Could you check a few things on this model? Use its own coordinates, in mm. Face numbers are marked on the shaded views. A direction names the side the tool comes from. Coordinates: 2 decimals unless noted, no trailing zeros. Loops run counter-clockwise (first coordinate to the right, second up) from the corner with the lowest first, then second, coordinate; pieces in that order, holes last. Notation, with made-up numbers: (67.25, 46.25) -> (107.25, 46.25) arc R19 ccw to (107.25, 81.25) -> close; hole circle Ø7 at (86.25, 87.5). An arc over 180 degrees is marked (long way). One line per question, with ' | ' between items.
Autodesk Inventor part; units mm, degrees
ref_plane "YZ Plane" through (0, 0, 0) normal (1, 0, 0) x (0, 1, 0)
ref_plane "XZ Plane" through (0, 0, 0) normal (0, 1, 0) x (-1, 0, 0)
ref_plane "XY Plane" through (0, 0, 0) normal (0, 0, 1) x (1, 0, 0)
sketch "Sketch1" plane through (0, 0, 0) normal (0, 0, 1) x (1, 0, 0)
  circle A0 centre (0, 0) radius 10
  arc A1 (21, 0) -> (-21, 0) centre (0, 0) ccw
  line L0 (0, 0) -> (0, -39) construction
  line L1 (0, -39) -> (21, -39)
  line L2 (0, -39) -> (-21, -39)
  line L3 (-21, -39) -> (-21, 0)
  line L4 (21, -39) -> (21, 0)
  dimension "d0" = 20
  dimension "d2" = 42
  dimension "d3" = 21
  dimension "d4" = 39
extrude "Extrusion1" add sketch "Sketch1" along normal mid plane 96
sketch "Sketch2" plane through (0, 0, 0) normal (0, 0, 1) x (1, 0, 0)
  circle A0 centre (0, 0) radius 10
  line L0 (-21, -39) -> (21, -39)
  line L1 (21, -39) -> (21, 0)
  arc A1 (21, 0) -> (-21, 0) centre (0, 0) ccw
  line L2 (-21, 0) -> (-21, -39)
  line L3 (-21, -36) -> (21, -36)
  line L4 (21, -36) -> (21, 0)
  line L5 (-21, -31.2069) -> (-21, 0)
  dimension "d7" = 3
extrude "Extrusion2" cut sketch "Sketch2" along normal mid plane 90 contours L2 A1 L1 L3
move or copy body "Move Body1" bodies to move or copy 1 copy no rotation origin (0, 0, 0) rotation axis (1, 0, 0) rotation angle 90
move or copy body "Move Body2" bodies to move or copy 1 copy no rotation origin (0, 0, 0) rotation axis (0, 0, 1) rotation angle 90
properties part number "Wrist_Roll"
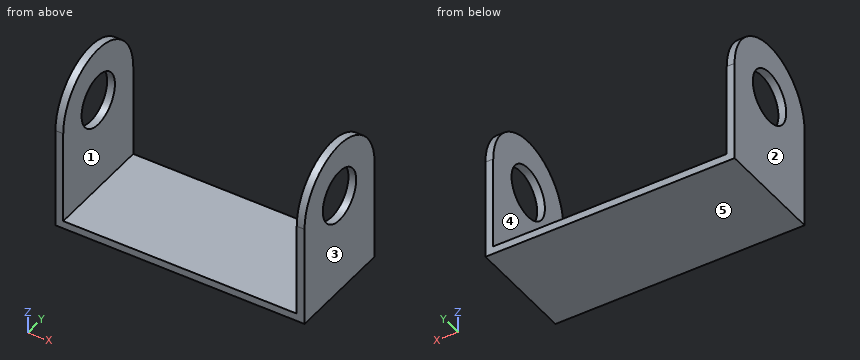
Q1. Imagine slicing it at D-D on x = -28.5. Write out the boundary of the cut face in (y, z).
Values follow:
outline: (-21, -39) -> (21, -39) -> (21, -36) -> (-21, -36) -> close
Q2. Imagine slicing it at A-A on z = -25.5. Write out the boundary of the cut face in (x, y).
Values follow:
outline: (-48, -21) -> (-45, -21) -> (-45, 21) -> (-48, 21) -> close; (45, -21) -> (48, -21) -> (48, 21) -> (45, 21) -> close
Q3. For pin 1 (4 mm diameter, centred on x = -28, y = 3, fed in from +Z), with a flat end and sliding along its axis, tell me the tip position at first contact or that it passes through.
Values follow:
pin 1: stops at z = -36
Q4. Imagine slicing it at C-C on z = -2. Write out the boundary of the cut face in (x, y).
Values follow:
outline: (-48, -21) -> (-45, -21) -> (-45, -9.8) -> (-48, -9.8) -> close; (-48, 9.8) -> (-45, 9.8) -> (-45, 21) -> (-48, 21) -> close; (45, -21) -> (48, -21) -> (48, -9.8) -> (45, -9.8) -> close; (45, 9.8) -> (48, 9.8) -> (48, 21) -> (45, 21) -> close
Q5. Imagine slicing it at B-B on y = 0. Write out the boundary of the cut face in (x, z), plus the area to 3 significant figures.
Values follow:
outline: (-48, -39) -> (48, -39) -> (48, -10) -> (45, -10) -> (45, -36) -> (-45, -36) -> (-45, -10) -> (-48, -10) -> close; (-48, 10) -> (-45, 10) -> (-45, 21) -> (-48, 21) -> close; (45, 10) -> (48, 10) -> (48, 21) -> (45, 21) -> close | area: 510 mm2
Q6. For the marked faces 1 and 2, which set-ups out of +Z, -Z, +X, -X, +Y, -Y let a thin tool reach every point of the face, with its end or its side?
Values follow:
face 1: +Z, +Y, -Y | face 2: +Z, -Z, -X, +Y, -Y
Q7. We'd pull the mould along X, two halves only. Please class the marked faces 3, 4 and 5: released by +X, released by -X, zero draft, split by the parting line, or undercut.
Values follow:
face 3: released by +X | face 4: undercut | face 5: zero draft
Q8. Please list where these lines run through material, in increasing order: L1, parallel to Z at x = 47, y = 0; L2, parallel to X at y = 5.5, z = -32.5; L3, parallel to Z at x = -24, y = -5. Write a range as [from, to].
Values follow:
L1: z = [-39, -10], [10, 21] | L2: x = [-48, -45], [45, 48] | L3: z = [-39, -36]
